```python
from build123d import *

# Parameters (mm, degrees)
SKETCH1_W             = 177.8
SKETCH1_H             = 114.3
SKETCH1_W_2           = 165.1
SKETCH1_H_2           = 16.134929366
BOSS_EXTRUDE1_DEPTH   = 1.524
CUT_EXTRUDE1_DEPTH    = 2.524
F_6_32_TAPPED_HOLE1_D = 2.7051
F_6_32_TAPPED_HOLE2_D = 2.7051


with BuildPart() as part:
    # Sketch1 → Boss-Extrude1 (new body)
    with BuildSketch(Plane(origin=(0, 0, 0), x_dir=(1, 0, 0), z_dir=(0, 1, 0))):
        Rectangle(SKETCH1_W, SKETCH1_H)
        with BuildLine():
            Line((-82.55, -25.4), (-82.55, -20.767464683))
            Line((-82.55, -20.767464683), (82.55, -20.767464683))
            Line((82.55, -20.767464683), (82.55, -25.4))
            ThreePointArc((82.55, -25.4), (64.589487758, -32.839487758), (57.15, -50.8))
            Line((57.15, -50.8), (-57.15, -50.8))
            ThreePointArc((-57.15, -50.8), (-64.589487758, -32.839487758), (-82.55, -25.4))
        make_face(mode=Mode.SUBTRACT)
        Rectangle(SKETCH1_W_2, SKETCH1_H_2, mode=Mode.SUBTRACT)
        with BuildLine():
            Line((82.55, 20.767464683), (-82.55, 20.767464683))
            Line((-82.55, 20.767464683), (-82.55, 25.4))
            ThreePointArc((-82.55, 25.4), (-64.589487758, 32.839487758), (-57.15, 50.8))
            Line((-57.15, 50.8), (57.15, 50.8))
            ThreePointArc((57.15, 50.8), (64.589487758, 32.839487758), (82.55, 25.4))
            Line((82.55, 25.4), (82.55, 20.767464683))
        make_face(mode=Mode.SUBTRACT)
    extrude(amount=BOSS_EXTRUDE1_DEPTH)

    # Sketch3 → Cut-Extrude1 (cut, through all)
    with BuildSketch(Plane(origin=(0, 1.524, 0), x_dir=(1, 0, 0), z_dir=(0, 1, 0))):
        with BuildLine():
            Line((-73.406, 16.004964683), (73.406, 16.004964683))
            ThreePointArc((73.406, 16.004964683), (74.9935, 14.417464683), (73.406, 12.829964683))
            Line((73.406, 12.829964683), (-73.406, 12.829964683))
            ThreePointArc((-73.406, 12.829964683), (-74.9935, 14.417464683), (-73.406, 16.004964683))
        make_face()
        with BuildLine():
            Line((-73.406, -16.004964683), (73.406, -16.004964683))
            ThreePointArc((73.406, -16.004964683), (74.9935, -14.417464683), (73.406, -12.829964683))
            Line((73.406, -12.829964683), (-73.406, -12.829964683))
            ThreePointArc((-73.406, -12.829964683), (-74.9935, -14.417464683), (-73.406, -16.004964683))
        make_face()
    extrude(amount=-CUT_EXTRUDE1_DEPTH, mode=Mode.SUBTRACT)

    # #6-32 Tapped Hole1 (through all)
    with Locations(Plane(origin=(0, 7.8105, 0), x_dir=(-1, 0, 0), z_dir=(0, 1, 0))):
        with Locations((82.55, -50.8), (82.55, 50.8), (-82.55, 50.8), (-82.55, -50.8)):
            Hole(F_6_32_TAPPED_HOLE1_D / 2)

    # #6-32 Tapped Hole2 (through all)
    with Locations(Plane(origin=(0, 1.524, 0), x_dir=(-1, 0, 0), z_dir=(0, 1, 0))):
        with Locations((82.55, -50.8), (82.55, 50.8), (-82.55, 50.8), (-82.55, -50.8)):
            Hole(F_6_32_TAPPED_HOLE2_D / 2)


solid = part.part
```
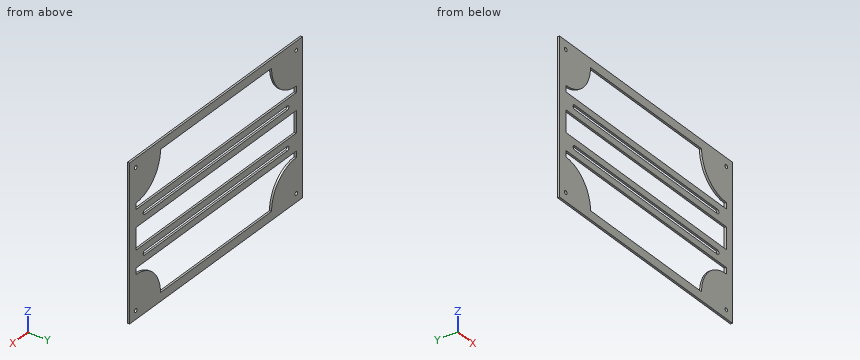
Geometry: final body of the model. Coordinates: model frame, mm. Round coordinates to 2 decimals unless told otherwise and drop trailing zeros. Order: outer loops, then holes, each group sorted by start corner. A loop starts at its lowest first (then second) coordinate and runs counter-clockwise, first axis right, second up. Notation, with made-up numbers: (22.25, 87.25) - (40.25, 87.25) arc R17 cw to (40.25, 98.25) - close; hole circle Ø6 at (37.25, -17.5). An arc over 180 degrees is marked (long way). Use CSV: the item, a comma, the result in double quotes. Start each with the question number.
Q1. Section query A-A (z = 23). Return loops of the section in (x, y).
Q2. Section query C-C (z = -33.5). Return loops of the section in (x, y), and give its area (3 significant figures).
Q3. Material intervals for line 1 along Z through (x, y) = (-47, 0.8); line 2 along X through (y, z) = (1.1, -3); line 3 along Z through (x, y) = (-71.5, 1.3), sorted ascending. Write a range as from..to.
Q4. Section query B-B (y = 0.3). State how many separate pieces and enclosed holes the cut face has, and give its area (3 significant figures).
Result set:
1,outline,"(-88.9, 0) - (-82.55, 0) - (-82.55, 1.52) - (-88.9, 1.52) - close; (82.55, 0) - (88.9, 0) - (88.9, 1.52) - (82.55, 1.52) - close"
2,outline,"(-88.9, 0) - (-63.95, 0) - (-63.95, 1.52) - (-88.9, 1.52) - close; (63.95, 0) - (88.9, 0) - (88.9, 1.52) - (63.95, 1.52) - close"
2,area,"76.0 mm2"
3,line 1,"z = -57.15..-50.8, -20.77..-16, -12.83..-8.07, 8.07..12.83, 16..20.77, 50.8..57.15"
3,line 2,"x = -88.9..-82.55, 82.55..88.9"
3,line 3,"z = -57.15..-27.93, -20.77..-16, -12.83..-8.07, 8.07..12.83, 16..20.77, 27.93..57.15"
4,separate pieces,"1"
4,enclosed holes,"9"
4,area,"8,800 mm2"
